from build123d import *

# Parameters (mm, degrees)
F0_R     = 2.3
F1_DEPTH = 5


with BuildPart() as f1:
    # F0 (on Top) → F1 (new body)
    with BuildSketch(Plane.XY):
        with BuildLine():
            Line((4, 42.95), (0, 42.95))
            Line((0, 42.95), (-2, 42.95))
            Line((-2, 42.95), (-2, 33.7))
            Line((-2, 33.7), (0, 33.7))
            Line((0, 33.7), (0, 0))
            Line((0, 0), (22.8, 0))
            Line((22.8, 0), (22.8, 33.7))
            Line((22.8, 33.7), (24.8, 33.7))
            Line((24.8, 33.7), (24.8, 42.95))
            Line((24.8, 42.95), (22.8, 42.95))
            Line((22.8, 42.95), (18.8, 42.95))
            Line((18.8, 42.95), (14.492329, 39.95))
            ThreePointArc((14.492329, 39.95), (11.4, 35.7), (8.307671, 39.95))
            Line((8.307671, 39.95), (4, 42.95))
        make_face()
        with Locations((11.4, 6.3)):
            Circle(F0_R, mode=Mode.SUBTRACT)
        with Locations((11.4, 19)):
            Circle(F0_R, mode=Mode.SUBTRACT)
    extrude(amount=F1_DEPTH)


solid = f1.part
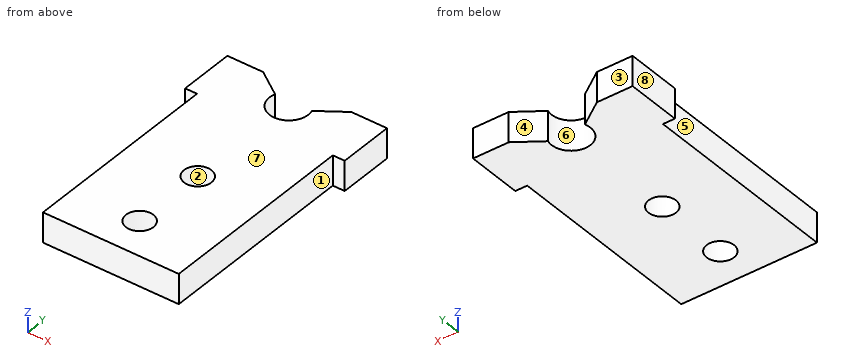
Source: CAD feature listing. Evaluate the final solid. Frame: model axes, mm. Face numbers are marked on the shaded views. A direction names the side the tool comes from. Round coordinates to 2 decimals unless told otherwise and drop trailing zeros. Loops run counter-clockwise (first coordinate to the right, second up) from the corner with the lowest first, then second, coordinate; pieces in that order, holes last. Notation, with made-up numbers: (-35.5, -19.5) -> (11.5, -19.5) arc R18 cw to (11.5, 5.5) -> close; hole circle Ø3 at (48, 12.25). An arc over 180 degrees is marked (long way). Answer as a JSON object with one key per item and string values. Group by question number.
Q1. Mould query, pull axis X, two halves, no side actions, for the marked faces 6, 7 and 8. Classes: pulls with the +X half, pulls with the -X half, needs draft (parallel to the pull), parting line crosses it, or undercut.
Q2. Section query B-B (x = 11.4). Output: boundary loops of the cut face in (y, z).
Q3. Contact query for flat-ended pins moving along their axis: P1, Ø1.5, axis at y = 15.5, z = 2, coming from the +X side; P2, Ø1.5, axis at y = 14, z = 1.5, coming from the -X side; P3, Ø2, axis at x = -1.5, z = 1.5, coming from the -Y side; P4, Ø4, axis at x = 11.4, y = 38.95, coming from the +Z side. Output: stop coordinate, or through.
Q4. Section query A-A (y = 38.95). Output: boundary loops of the cut face in (x, z).
Q5. Section query D-D (y = 6.3). Output: boundary loops of the cut face in (x, z), plus the area to 3 significant figures.
Q6. Ray query, line 1 (Y direction, x = 11.4, z = 1.45); line 2 (Y direction, x = 10.25, z = 0.35); line 3 (X direction, y = 16.5, z = 4.5). Return the intervals inside material, ascending. Write a range as from..to.
Q7. Access query for the marked faces 1, 2, 3, 4 and 5. Directions: +Z, -Z, +X, -X, +Y, -Y. A direction counts if a zero-diameter tool reaches every point of the face in a straight line with its end or side. Return the directions, or none.
Q8. Section query C-C (z = 0.85). Output: boundary loops of the cut face in (x, y).
Completed:
{
 "1": {"face 6": "undercut", "face 7": "needs draft", "face 8": "pulls with the -X half"},
 "2": {"outline": "(0, 0) -> (4, 0) -> (4, 5) -> (0, 5) -> close; (8.6, 0) -> (16.7, 0) -> (16.7, 5) -> (8.6, 5) -> close; (21.3, 0) -> (35.7, 0) -> (35.7, 5) -> (21.3, 5) -> close"},
 "3": {"P1": "x = 22.8", "P2": "x = 0", "P3": "y = 33.7", "P4": "through"},
 "4": {"outline": "(-2, 0) -> (8.15, 0) -> (8.15, 5) -> (-2, 5) -> close; (14.65, 0) -> (24.8, 0) -> (24.8, 5) -> (14.65, 5) -> close"},
 "5": {"outline": "(0, 0) -> (9.1, 0) -> (9.1, 5) -> (0, 5) -> close; (13.7, 0) -> (22.8, 0) -> (22.8, 5) -> (13.7, 5) -> close", "area": "91.0 mm²"},
 "6": {"line 1": "0..4, 8.6..16.7, 21.3..35.7", "line 2": "0..4.31, 8.29..17.01, 20.99..35.91", "line 3": "0..22.8"},
 "7": {"face 1": "+Z, -Z, +X, -Y", "face 2": "+Z, -Z", "face 3": "+Z, -Z, +X, -X, +Y", "face 4": "+Z, -Z, +Y", "face 5": "+Z, -Z, -X, -Y"},
 "8": {"outline": "(-2, 33.7) -> (0, 33.7) -> (0, 0) -> (22.8, 0) -> (22.8, 33.7) -> (24.8, 33.7) -> (24.8, 42.95) -> (18.8, 42.95) -> (14.49, 39.95) arc R3.25 cw (long way) to (8.31, 39.95) -> (4, 42.95) -> (-2, 42.95) -> close; hole circle Ø4.6 at (11.4, 6.3); hole circle Ø4.6 at (11.4, 19)"}
}
